The figure shows three views and two pictorial views of one solid part (mm, origin at its lowest corner). Answer the questions. A direction names the side the tool comes from. Coordinates: 2 decimals unless noted, no trailing zeros. Order: outer loops, then holes, each group sorted by start corner. A loop starts at its lowest first (then second) coordinate and runs counter-clockwise, first axis right, second up. Notation, with made-up numbers: (29.5, -17.5) - (44.5, -17.5) arc R19 ccw to (44.5, 7.5) - close; hole circle Ø2 at (13.25, 46.25). An arc over 180 degrees is marked (long way). Use one line per item in the form item = value. Start each with the question number.
Item 1: Section B-B, the plane x = 3 is taken. Write down the section's boundary in (y, z).
Item 2: Each of these flat-tipped pins is pushed along its axis until it touches: pin 1 Ø10 at (x, y) = (8, 7) entering from -Z; pin 2 Ø0.9 at (y, z) = (2, 1) entering from -X; pin 3 Ø0.9 at (x, z) = (2, 1) entering from -Y; pin 4 Ø0.9 at (y, z) = (2, 1.5) entering from +X. Where does it stop, or does it pass through?
Item 3: Consider line 1 along Y through (x, z) = (16.5, 2.1); line 2 along Y through (x, z) = (2.75, 1.3); line 3 along X through (y, z) = (53, 2.2). Determine where each line is inside the solid, lowest interval first. Write a range as [from, to].
Item 4: Section C-C, the plane x = 11.25 is taken. Write down the section's boundary in (y, z), and give its area (4 significant figures).
Item 5: Section A-A, the plane z = 0.95 is taken. Write down the section's boundary in (x, y).
Item 6: A tool of negligible diameter and unlimited length cuts with its end or side. For the marked faces 1, 2, 3, 4 and 5, from which of +Z, -Z, +X, -X, +Y, -Y can it reach the whole face along a straight path? Write none if from no direction.
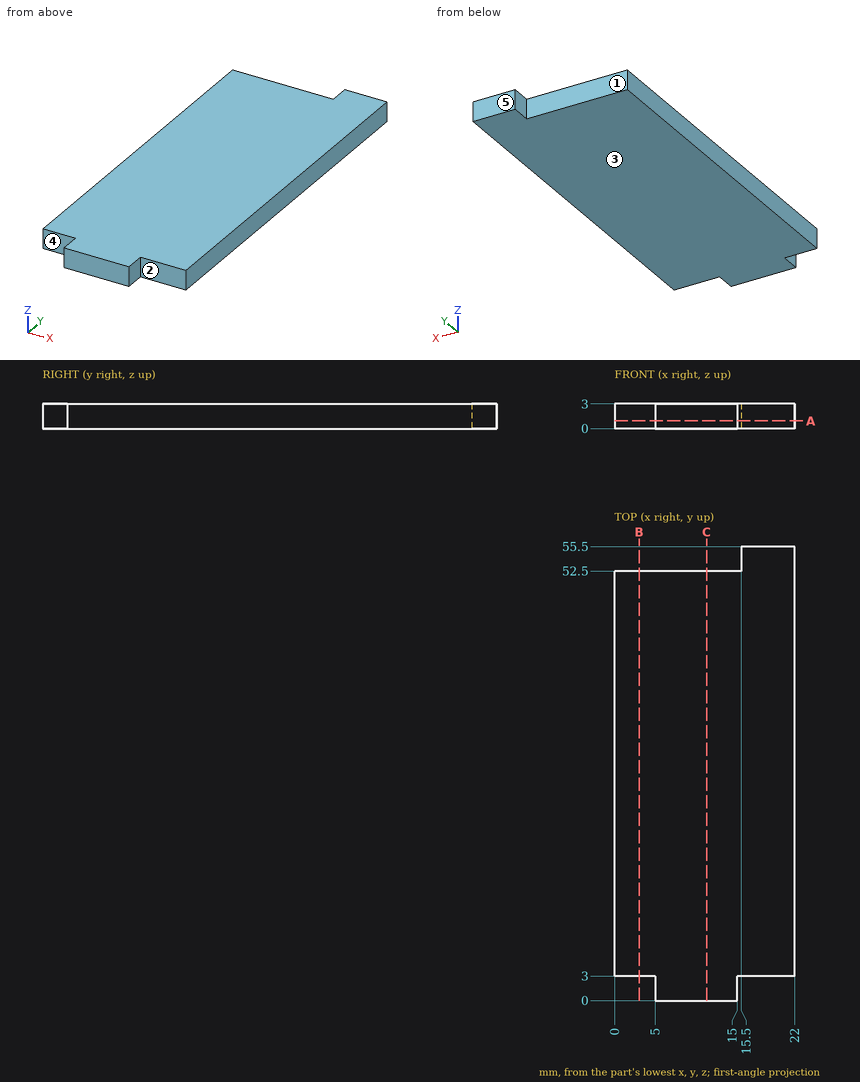
Response:
q1.outline = (3, 0) - (52.5, 0) - (52.5, 3) - (3, 3) - close
q2.pin_1 = 0
q2.pin_2 = 5
q2.pin_3 = 3
q2.pin_4 = 15
q3.line_1 = [3, 55.5]
q3.line_2 = [3, 52.5]
q3.line_3 = [15.5, 22]
q4.outline = (0, 0) - (52.5, 0) - (52.5, 3) - (0, 3) - close
q4.area = 157.5 mm2
q5.outline = (0, 3) - (5, 3) - (5, 0) - (15, 0) - (15, 3) - (22, 3) - (22, 55.5) - (15.5, 55.5) - (15.5, 52.5) - (0, 52.5) - close
q6.face_1 = +Z, -Z, -X, +Y
q6.face_2 = +Z, -Z, +X, -Y
q6.face_3 = -Z, +X, -X, +Y, -Y
q6.face_4 = +Z, -Z, -X, -Y
q6.face_5 = +Z, -Z, +X, -X, +Y
